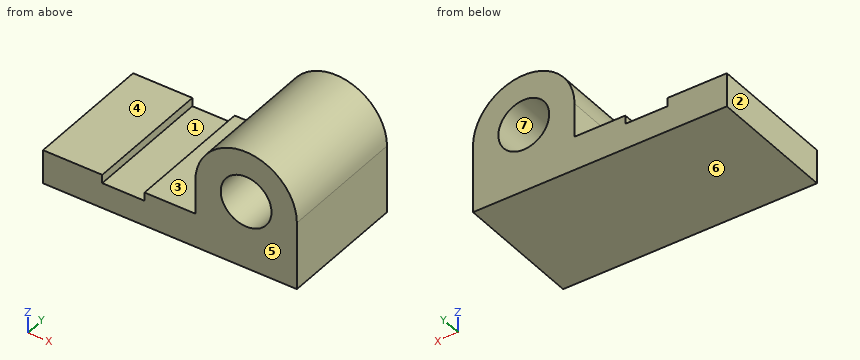
```python
from build123d import *

# Parameters (mm, degrees)
F0_R     = 15
F1_DEPTH = 76.2


with BuildPart() as f1:
    # F0 (on Front) → F1 (new body)
    with BuildSketch(Plane.XZ):
        with BuildLine():
            Line((0, 20), (0, 0))
            Line((0, 0), (150, 0))
            Line((150, 0), (150, 40))
            ThreePointArc((150, 40), (120, 70), (90, 40))
            Line((90, 40), (90, 20))
            Line((90, 20), (60, 20))
            Line((60, 20), (60, 15))
            Line((60, 15), (35, 15))
            Line((35, 15), (35, 20))
            Line((35, 20), (0, 20))
        make_face()
        with Locations((120, 40)):
            Circle(F0_R, mode=Mode.SUBTRACT)
    extrude(amount=F1_DEPTH)


solid = f1.part
```
Model file for the job. Use its own axes, mm. Face numbers are marked on the shaded views. A direction names the side the tool comes from. Round coordinates to 2 decimals unless told otherwise and drop trailing zeros. Write each loop counter-clockwise with the first axis right and the second up, starting at its lowest first coordinate (ties: lowest second). Pieces come first, ordered by that corner, then holes. Notation, with made-up numbers: (-21.75, 33) - (24.25, 33) arc R20 ccw to (24.25, 46) - close; hole circle Ø11 at (-9, -28). An arc over 180 degrees is marked (long way). Use CSV: the item, a comma, the result in double quotes. Start each with the question number.
Item 1: Drill centre lines: L1, parallel to X at y = -25.5, z = 17.5; L2, parallel to Z at x = 120, y = -53; L3, parallel to Z at x = 116, y = -19. Where is each one in solid material? Low to high. Write a range as [from, to].
Item 2: Band-saw the part on B-B (z = 47.5). Write the cut outline in (x, y), and give its area (3 significant figures).
Item 3: Band-saw the part on D-D (z = 58.5). Write the cut outline in (x, y).
Item 4: Pin check, flat tips, straight feed: P1, Ø17.5, axis at x = 16, y = -47, coming from the +Z side; P2, Ø8, axis at y = -67, z = 33, coming from the -X side; P3, Ø6, axis at x = 124, y = -19, coming from the -Z side; P4, Ø8, axis at y = -60.5, z = 60.5, coming from the -X side. Stop position of each tip, or through.
Item 5: Two-plate mould, pull along Z, no slides. Class the marked faces 4, 5, 6 and 7: released by +Z, released by -Z, zero draft, split by the parting line, or undercut.
Item 6: Tool access for the marked faces 1, 2 and 3: list every direction of +Z, -Z, +X, -X, +Y, -Y with a clear straight run to the whole face (end or side of a thin tool).
Item 7: Band-saw the part on C-C (y = -58). Write the cut outline in (x, z).
Item 8: Band-saw the part on A-A (x = 120). Write the cut outline in (y, z), and give its area (3 significant figures).
Checked values:
1,L1,"x = [0, 35], [60, 150]"
1,L2,"z = [0, 25], [55, 70]"
1,L3,"z = [0, 25.54], [54.46, 69.73]"
2,outline,"(90.95, -76.2) - (107.01, -76.2) - (107.01, 0) - (90.95, 0) - close; (132.99, -76.2) - (149.05, -76.2) - (149.05, 0) - (132.99, 0) - close"
2,area,"2,450 mm²"
3,outline,"(96.38, -76.2) - (143.62, -76.2) - (143.62, 0) - (96.38, 0) - close"
4,P1,"stops at z = 20"
4,P2,"stops at x = 90"
4,P3,"stops at z = 0"
4,P4,"stops at x = 94.95"
5,face 4,"released by +Z"
5,face 5,"zero draft"
5,face 6,"released by -Z"
5,face 7,"undercut"
6,face 1,"+Z, +Y, -Y"
6,face 2,"+Z, -Z, -X, +Y, -Y"
6,face 3,"+Z, -X, +Y, -Y"
7,outline,"(0, 0) - (150, 0) - (150, 40) arc R30 ccw to (90, 40) - (90, 20) - (60, 20) - (60, 15) - (35, 15) - (35, 20) - (0, 20) - close; hole circle Ø30 at (120, 40)"
8,outline,"(-76.2, 0) - (0, 0) - (0, 25) - (-76.2, 25) - close; (-76.2, 55) - (0, 55) - (0, 70) - (-76.2, 70) - close"
8,area,"3,050 mm²"
